The model under review builds one solid part; all positions refer to its coordinate system, in mm. A direction names the side the tool comes from. Coordinates: 2 decimals unless noted, no trailing zeros. Order: outer loops, then holes, each group sorted by start corner. A loop starts at its lowest first (then second) coordinate and runs counter-clockwise, first axis right, second up. Notation, with made-up numbers: M 19,-1.75 L 29,-1.75 A9 ccw 29,6.25 Z; hole C -34.5,22 d5. An arc over 180 degrees is marked long. Answer as CSV lines item,"result". Start each with the question number.
Q1. Consider section D-D on z = 976.5. Write out the cut boundary in (x, y).
Q2. For P1, Ø1.5, axis at x = -9.5, z = 384.5, coming from the +Y side; P2, Ø7, axis at y = 29.5, z = 15.5, coming from the -X side; P3, Ø4, axis at x = -24.5, z = 515, coming from the -Y side; P4, Ø6, axis at x = -21.5, y = -24.5, coming from the -Z side, all flat-tipped, find the tip position at first contact; note any pin that passes through.
Q3. Wall thickness on L1, parallel to Y at x = -0.5, z = 88; L2, parallel to Z at x = 16.5, y = -7.5: over which ranges is each line inside the solid? List them lowest first. Write a range as [from, to].
Q4. Machinability: for faces 4 (the face through (21, -21, 0)), 5 (the face through (0, 0, 609.6)), which of the approach directions +Z, -Z, +X, -X, +Y, -Y give a long, thin tool a straight path to every point of the face, cutting with its end or side? Answer none if there is none.
Q5. Consider section B-B on z = 569. Write out the cut boundary in (x, y), and give its area (3 significant figures).
Q6. The part is to be moulded in two halves that separate along Y. For faces 1 (the face through (-30.235, -23.183, 594.84)), 2 (the face through (-21, 21, 0)), 3 (the face through (5.506, -24.796, 300.533)), say which applies: +Y half, -Y half, draft (parallel to the pull), parting line (faces both ways), or undercut.
Q7. Consider section A-A on x = 0. Write out the cut boundary in (y, z), and give its area (3 significant figures).
from build123d import *

# Parameters (mm, degrees)
SKETCH1_R           = 38.1
BOSS_EXTRUDE1_DEPTH = 1206.5
FILLET1_R           = 2.54
FILLET2_R           = 2.54
CUT_EXTRUDE2_DEPTH  = 25.4
SKETCH2_R           = 25.4
CUT_EXTRUDE1_DEPTH  = 609.6


with BuildPart() as part:
    # Sketch1 → Boss-Extrude1 (new body)
    with BuildSketch(Plane.XY):
        Circle(SKETCH1_R)
    extrude(amount=BOSS_EXTRUDE1_DEPTH)

    # Fillet1
    fillet1_edges = [part.edges().sort_by_distance(p)[0] for p in [
        (-38.1, 0, 1206.5),
    ]]
    fillet(fillet1_edges, radius=FILLET1_R)

    # Fillet2
    fillet2_edges = [part.edges().sort_by_distance(p)[0] for p in [
        (-38.1, 0, 0),
    ]]
    fillet(fillet2_edges, radius=FILLET2_R)

    # Sketch3 → Cut-Extrude2 (cut)
    with BuildSketch(Plane(origin=(0, 0, 0), x_dir=(-1, 0, 0), z_dir=(0, 0, -1))):
        Polygon((12.7, 12.7), (64.136774618, 12.7), (64.136774618, -12.7), (12.7, -12.7), (12.7, -42.915047722), (-12.7, -42.915047722), (-12.7, -12.7), (-64.765566526, -12.7), (-64.765566526, 12.7), (-12.7, 12.7), (-12.7, 40.714276044), (12.7, 40.714276044), align=None)
    extrude(amount=-CUT_EXTRUDE2_DEPTH, mode=Mode.SUBTRACT)

    # Sketch2 → Cut-Extrude1 (cut)
    with BuildSketch(Plane(origin=(0, 0, 0), x_dir=(-1, 0, 0), z_dir=(0, 0, -1))):
        Circle(SKETCH2_R)
    extrude(amount=-CUT_EXTRUDE1_DEPTH, mode=Mode.SUBTRACT)


solid = part.part
Evaluation:
1,outline,"C 0,0 d76.2"
2,P1,"stops at y = 37.08"
2,P2,"stops at x = -27.85"
2,P3,"stops at y = -30.75"
2,P4,"stops at z = 0"
3,L1,"y = [-38.1, -25.4], [25.4, 38.1]"
3,L2,"z = [609.6, 1206.5]"
4,face 4,"-Z, +X, -X, +Y, -Y"
4,face 5,"-Z"
5,outline,"C 0,0 d76.2; hole C 0,0 d50.8"
5,area,"2,530 mm²"
6,face 1,"parting line"
6,face 2,"draft"
6,face 3,"undercut"
7,outline,"M -38.1,25.4 L -25.4,25.4 L -25.4,609.6 L 25.4,609.6 L 25.4,25.4 L 38.1,25.4 L 38.1,1203.96 A2.54 ccw 35.56,1206.5 L -35.56,1206.5 A2.54 ccw -38.1,1203.96 Z"
7,area,"60,300 mm²"
